Work out the finished part from the listing and answer in its coordinate system (mm). Face numbers are marked on the shaded views. A direction names the side the tool comes from. Give positions to 0.01 mm unless a question says otherwise; leave off trailing zeros. Write each loop counter-clockwise with the first axis right and the second up, starting at its lowest first coordinate (ties: lowest second). Pieces come first, ordered by that corner, then holes.
1) Find section C-C (y = 0.5). Determine the outline of the cut face in (x, z).
2) Find section D-D (z = 5.5). Determine the outline of the cut face in (x, y).
3) Find section A-A (x = 0). Determine the outline of the cut face in (y, z), plus the area to 3 significant figures.
4) Straight lines are drawn through the part: probe 1 along Z at (x, y) = (0, 3.3); probe 2 along Z at (x, y) = (0, 5.7); probe 3 along Y at (x, z) = (-3.5, 3.5). For each, find the intervals that lie inside material, in ascending order.
5) A tool of negligible diameter and unlimited length cuts with its end or side. For the marked faces 1 and 2, from which of +Z, -Z, +X, -X, +Y, -Y can it reach the whole face along a straight path? Write none if from no direction.
6) Determine the mould class of the marked faces 3, 4, 5 and 6 for opening direction Z: pulls with the +Z half, pulls with the -Z half, needs draft (parallel to the pull), parting line crosses it, or undercut.
7) Given pin 1 Ø3 at (x, z) = (0, 14) entering from -Y; pin 2 Ø2 at (x, z) = (-1, -4) entering from -Y; pin 3 Ø1.5 at (x, y) = (6.5, 4.5) entering from +Z; pin 4 Ø1 at (y, z) = (2.5, 12) entering from +X, each flat-ended and moving along its own axis, determine where each tip first touches the part or whether it passes through.
8) Find section B-B (z = 0). Determine the outline of the cut face in (x, y).
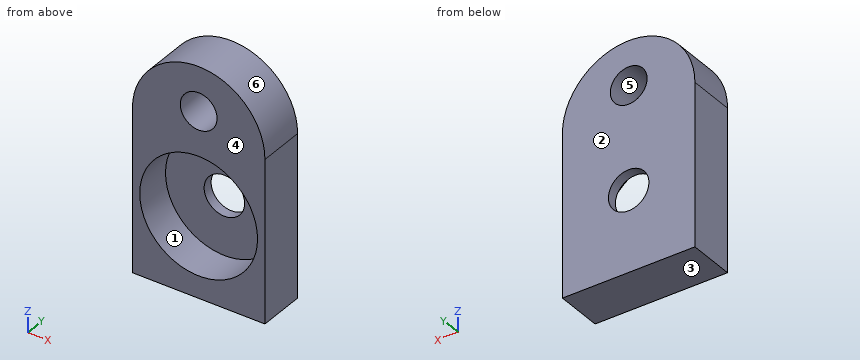
```python
from build123d import *

# Parameters (mm, degrees)
BOSS_EXTRUDE1_DEPTH = 6.35
SKETCH2_R           = 8
CUT_EXTRUDE1_DEPTH  = 5
SKETCH3_R           = 2.75
CUT_EXTRUDE2_DEPTH  = 2.35
SKETCH4_R           = 2.5
CUT_EXTRUDE3_DEPTH  = 7.35


with BuildPart() as part:
    # Sketch1 → Boss-Extrude1 (new body)
    with BuildSketch(Plane(origin=(0, 0, 0), x_dir=(1, 0, 0), z_dir=(0, 1, 0))):
        with BuildLine():
            Line((9, 11), (-9, 11))
            Line((-9, 11), (-9, -11))
            ThreePointArc((-9, -11), (0, -20), (9, -11))
            Line((9, -11), (9, 11))
        make_face()
    extrude(amount=BOSS_EXTRUDE1_DEPTH)

    # Sketch2 → Cut-Extrude1 (cut)
    with BuildSketch(Plane.XZ):
        Circle(SKETCH2_R)
    extrude(amount=-CUT_EXTRUDE1_DEPTH, mode=Mode.SUBTRACT)

    # Sketch3 → Cut-Extrude2 (cut, through all)
    with BuildSketch(Plane.XZ.offset(-5)):
        Circle(SKETCH3_R)
    extrude(amount=-CUT_EXTRUDE2_DEPTH, mode=Mode.SUBTRACT)

    # Sketch4 → Cut-Extrude3 (cut, through all)
    with BuildSketch(Plane.XZ):
        with Locations((0, 14)):
            Circle(SKETCH4_R)
        with Locations((0, -13.5)):
            Circle(SKETCH4_R)
    extrude(amount=-CUT_EXTRUDE3_DEPTH, mode=Mode.SUBTRACT)


solid = part.part
```
Results:
1. outline: (-9, -11) - (9, -11) - (9, 11) arc R9 ccw to (-9, 11) - close; hole circle Ø16 at (0, 0); hole circle Ø5 at (0, 14)
2. outline: (-9, 0) - (-5.81, 0) - (-5.81, 5) - (5.81, 5) - (5.81, 0) - (9, 0) - (9, 6.35) - (-9, 6.35) - close
3. outline: (0, -11) - (6.35, -11) - (6.35, -2.75) - (5, -2.75) - (5, -8) - (0, -8) - close; (0, 8) - (5, 8) - (5, 2.75) - (6.35, 2.75) - (6.35, 11.5) - (0, 11.5) - close; (0, 16.5) - (6.35, 16.5) - (6.35, 20) - (0, 20) - close
3. area: 77.7 mm2
4. probe 1: z = -11 to -8, 8 to 11.5, 16.5 to 20
4. probe 2: z = -11 to -2.75, 2.75 to 11.5, 16.5 to 20
4. probe 3: y = 5 to 6.35
5. face 1: -Y
5. face 2: +Z, -Z, +X, -X, +Y
6. face 3: pulls with the -Z half
6. face 4: needs draft
6. face 5: undercut
6. face 6: pulls with the +Z half
7. pin 1: passes through
7. pin 2: stops at y = 5
7. pin 3: stops at z = 17.92
7. pin 4: stops at x = 8.99
8. outline: (-9, 0) - (-8, 0) - (-8, 5) - (-2.75, 5) - (-2.75, 6.35) - (-9, 6.35) - close; (2.75, 5) - (8, 5) - (8, 0) - (9, 0) - (9, 6.35) - (2.75, 6.35) - close
